Job drawing, mm, ordinate dimensions from the low corner. One solid piece. Give positions to 0.01 mm unless a question says otherwise; leave off trailing zeros. Write each loop counter-clockwise with the first axis right and the second up, starting at its lowest first coordinate (ties: lowest second). Pieces come first, ordered by that corner, then holes. Notation, with made-up numbers: (82.5, 49) - (113.5, 49) arc R26 cw to (113.5, 82) - close; hole circle Ø4 at (-12, 52). An arc over 180 degrees is marked (long way). Put each result on its own line as item: value. Start each with the question number.
1. Cut at C-C on x = 2.35. List the corners of the cut face in (y, z).
2. Mould opens along Z. For the marked faces 1, 2 and 3 say: +Z half, -Z half, draft (parallel to the pull), parting line (faces both ways), or undercut.
3. Cut at A-A on x = 1.9. List the corners of the cut face in (y, z).
4. Cut at B-B on z = 6.75. List the corners of the cut face in (x, y).
5. Wall check: line 1 (Z direction, x = 0.8, y = 4.75); line 2 (Y direction, x = 1.4, z = 3.25) (1 decimal); line 3 (Z direction, x = 2.3, y = 7.75) (1 decimal). Give the ranges that are in metal, low to high.
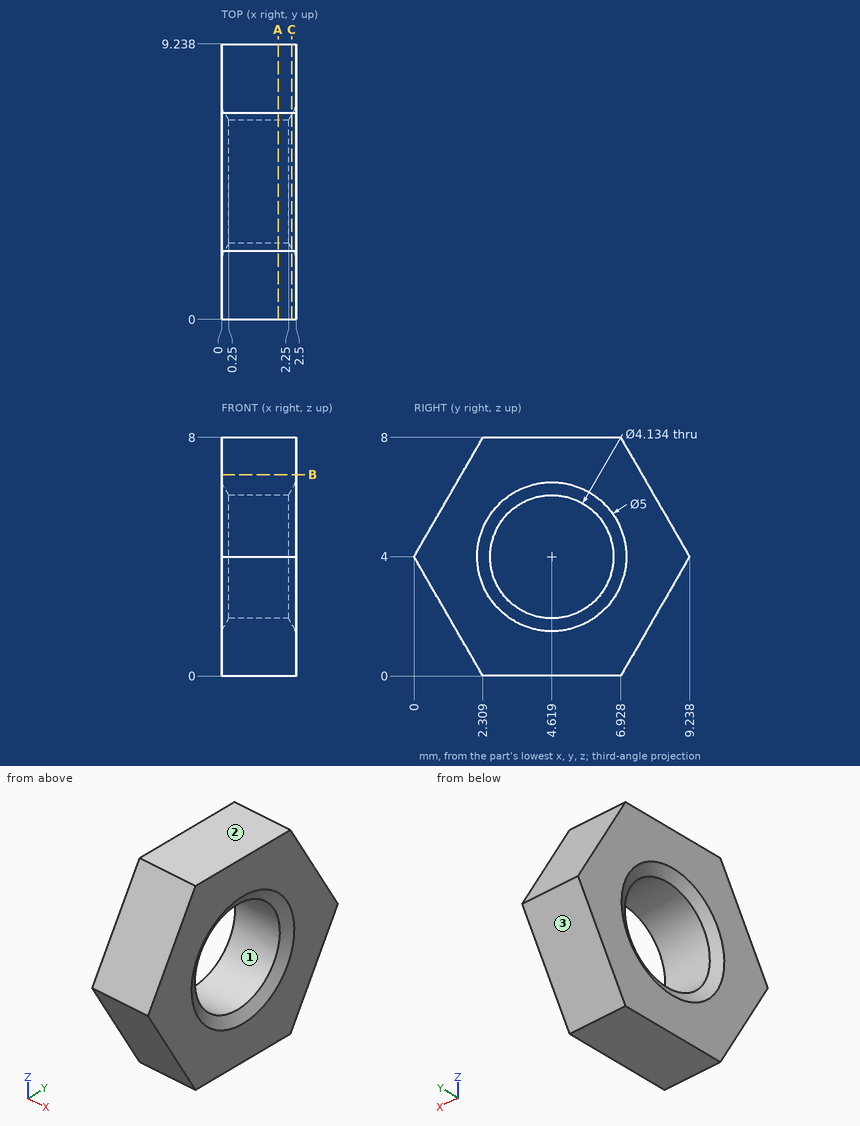
Report:
1. outline: (0, 4) - (2.31, 0) - (6.93, 0) - (9.24, 4) - (6.93, 8) - (2.31, 8) - close; hole circle Ø4.48 at (4.62, 4)
2. face 1: undercut
2. face 2: +Z half
2. face 3: -Z half
3. outline: (0, 4) - (2.31, 0) - (6.93, 0) - (9.24, 4) - (6.93, 8) - (2.31, 8) - close; hole circle Ø4.13 at (4.62, 4)
4. outline: (0, 1.59) - (2.5, 1.59) - (2.5, 7.65) - (0, 7.65) - close
5. line 1: z = 0 to 1.94, 6.06 to 8
5. line 2: y = 0.4 to 2.7, 6.5 to 8.8
5. line 3: z = 1.4 to 6.6
